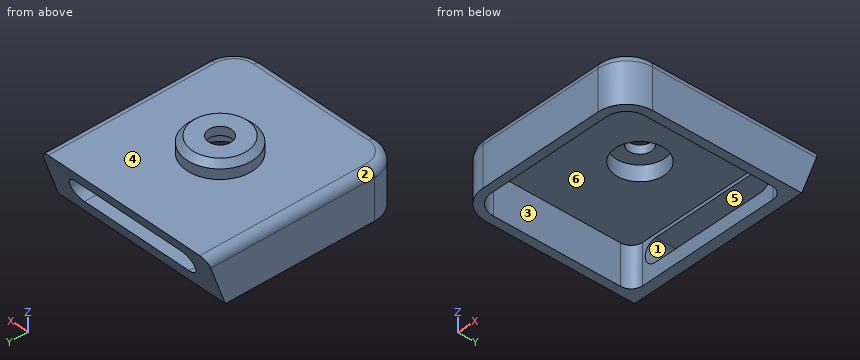
from build123d import *

# Parameters (mm, degrees)
SKETCH1_W           = 32
SKETCH1_H           = 31.091910702798558
BOSS_EXTRUDE1_DEPTH = 1.5
FILLET1_R           = 5
SKETCH2_R           = 4.3000000000159515
CUT_EXTRUDE1_DEPTH  = 45.642545975233084
SKETCH3_R           = 5.79999999998862
SKETCH3_R_2         = 4.299999999994187
BOSS_EXTRUDE2_DEPTH = 1.212999868
SKETCH4_R           = 5.799999999994187
SKETCH4_R_2         = 1.9999999999941904
BOSS_EXTRUDE3_DEPTH = 1.5
CHAMFER1_SIZE       = 1
EXTRUDE_THIN1_DEPTH = 7.05
BOSS_EXTRUDE4_REACH = 47.171
SKETCH7_W           = 29.000000000000004
SKETCH7_H           = 1.8000000000000007
BOSS_EXTRUDE5_DEPTH = 7.05
FILLET2_R           = 2
CUT_EXTRUDE2_DEPTH  = 10
FILLET3_R           = 1.5


with BuildPart() as part:
    # Sketch1 → Boss-Extrude1 (new body)
    with BuildSketch(Plane.XY):
        with Locations((16, 15.545955351399279)):
            Rectangle(SKETCH1_W, SKETCH1_H)
    extrude(amount=BOSS_EXTRUDE1_DEPTH)

    # Fillet1
    fillet1_edges = [part.edges().sort_by_distance(p)[0] for p in [
        (32, 0, 0.75),
        (0, 0, 0.75),
    ]]
    fillet(fillet1_edges, radius=FILLET1_R)

    # Sketch2 → Cut-Extrude1 (cut, through all)
    with BuildSketch(Plane(origin=(0, 0, 0), x_dir=(-1, 0, 0), z_dir=(0, 0, -1))):
        with Locations((-15.991678414180004, 17.403095514898066)):
            Circle(SKETCH2_R)
    extrude(amount=-CUT_EXTRUDE1_DEPTH, mode=Mode.SUBTRACT)

    # Sketch3 → Boss-Extrude2 (add)
    with BuildSketch(Plane.XY.offset(1.5)):
        with Locations(Location((15.991678414180004, 17.403095514898066, 0), (0, 0, 180))):
            Circle(SKETCH3_R)
        with Locations(Location((15.991678414180004, 17.403095514898066, 0), (0, 0, 180))):
            Circle(SKETCH3_R_2, mode=Mode.SUBTRACT)
    extrude(amount=BOSS_EXTRUDE2_DEPTH)

    # Sketch4 → Boss-Extrude3 (add)
    with BuildSketch(Plane.XY.offset(2.7129998678795)):
        with Locations(Location((15.991678414180004, 17.403095514898066, 0), (0, 0, 180))):
            Circle(SKETCH4_R)
        with Locations((15.991678414180004, 17.403095514898066)):
            Circle(SKETCH4_R_2, mode=Mode.SUBTRACT)
    extrude(amount=BOSS_EXTRUDE3_DEPTH)

    # Chamfer1
    chamfer1_edges = [part.edges().sort_by_distance(p)[0] for p in [
        (21.791678414174193, 17.403095514898062, 4.2129998678795),
    ]]
    chamfer(chamfer1_edges, length=CHAMFER1_SIZE)

    # Sketch5 → Extrude-Thin1 (add)
    with BuildSketch(Plane(origin=(0, 0, 0), x_dir=(-1, 0, 0), z_dir=(0, 0, -1))):
        with BuildLine():
            Line((0, 31.091910702798558), (0, 4.999999999999998))
            ThreePointArc((0, 4.999999999999998), (-1.4644660940672622, 1.4644660940672614), (-5, 0))
            Line((-5, 0), (-27, 0))
            ThreePointArc((-27, 0), (-30.535533905932738, 1.4644660940672654), (-32, 4.999999999999998))
            Line((-32, 4.999999999999998), (-32, 31.091910702798558))
            Line((-32, 31.091910702798558), (-30.5, 31.091910702798558))
            Line((-30.5, 31.091910702798558), (-30.5, 4.999999999999998))
            ThreePointArc((-30.5, 4.999999999999996), (-29.47487373415292, 2.5251262658470903), (-27.00000000000001, 1.5000000000000067))
            Line((-27, 1.5), (-5, 1.5))
            ThreePointArc((-4.999999999999999, 1.5), (-2.525126265847083, 2.5251262658470828), (-1.4999999999999996, 4.999999999999998))
            Line((-1.5, 4.999999999999998), (-1.5, 31.091910702798558))
            Line((-1.5, 31.091910702798558), (0, 31.091910702798558))
        make_face()
    extrude(amount=EXTRUDE_THIN1_DEPTH)

    # Boss-Extrude4: up to this face of the body (flat: up to its plane)
    boss_extrude4_end = Plane(part.part.faces().sort_by_distance((0, 18.045955351, -2.775))[0])
    # Sketch6 → Boss-Extrude4 (add, up to the picked face)
    with BuildSketch(Plane(origin=(32, 0, 0), x_dir=(0, 0, -1), z_dir=(1, 0, 0)), mode=Mode.PRIVATE) as boss_extrude4_sk1:
        Polygon((7.050000000000448, 31.09191070279875), (-1.4999999999999993, 34.20385620577456), (-1.5, 31.091910702798558), align=None)
    boss_extrude4_tool1 = split(extrude(boss_extrude4_sk1.sketch, amount=-BOSS_EXTRUDE4_REACH, mode=Mode.PRIVATE), bisect_by=boss_extrude4_end, keep=Keep.BOTH, mode=Mode.PRIVATE)
    add(boss_extrude4_tool1.solids().sort_by(Axis((32, 32.129226, -1.35), (-1, 0, 0)))[0])

    # Sketch7 → Boss-Extrude5 (add)
    with BuildSketch(Plane(origin=(0, 0, 0), x_dir=(-1, 0, 0), z_dir=(0, 0, -1))):
        with Locations((-16, 30.19191070279856)):
            Rectangle(SKETCH7_W, SKETCH7_H)
    extrude(amount=BOSS_EXTRUDE5_DEPTH)

    # Fillet2
    fillet2_edges = [part.edges().sort_by_distance(p)[0] for p in [
        (30.5, 29.291910702798557, -3.525),
        (1.5, 29.291910702798557, -3.525),
    ]]
    fillet(fillet2_edges, radius=FILLET2_R)

    # Sketch8 → Cut-Extrude2 (cut)
    with BuildSketch(Plane.XZ.offset(-29.291910702798557)):
        with BuildLine():
            Line((26, -4.600000000000001), (6.000000000000002, -4.600000000000004))
            ThreePointArc((6.000000000000002, -4.600000000000004), (3.9999999999999996, -2.600000000000004), (6.000000000000001, -0.6000000000000024))
            Line((6.000000000000001, -0.6000000000000024), (26, -0.6))
            ThreePointArc((26, -0.6), (28, -2.600000000000002), (26, -4.600000000000001))
        make_face()
    extrude(amount=-CUT_EXTRUDE2_DEPTH, mode=Mode.SUBTRACT)

    # Fillet3
    fillet3_edges = [part.edges().sort_by_distance(p)[0] for p in [
        (32, 19.60192810288728, 1.4999999999999996),
        (16, 0, 1.5),
        (1.4644660940672618, 1.4644660940672614, 1.5),
        (30.535533905932738, 1.4644660940672618, 1.5),
        (-4.4e-16, 19.60192810288728, 1.4999999999999996),
    ]]
    fillet(fillet3_edges, radius=FILLET3_R)


solid = part.part
The model under review builds one solid part; all positions refer to its coordinate system, in mm. Face numbers are marked on the shaded views. A direction names the side the tool comes from. Coordinates: 2 decimals unless noted, no trailing zeros. Order: outer loops, then holes, each group sorted by start corner. A loop starts at its lowest first (then second) coordinate and runs counter-clockwise, first axis right, second up. Notation, with made-up numbers: (-30, -6.5) -> (21, -6.5) arc R18 cw to (21, 9.5) -> close; hole circle Ø7 at (20.25, 33.25). An arc over 180 degrees is marked (long way). Answer in a Markdown table with one row per item.
(1) Consider section B-B (y = 26). Write out the cut boundary in (x, z).
Answers:
| item | result |
|---|---|
| outline | (0, -7.05) -> (1.5, -7.05) -> (1.5, 0) -> (30.5, 0) -> (30.5, -7.05) -> (32, -7.05) -> (32, 0) arc R1.5 ccw to (30.5, 1.5) -> (1.5, 1.5) arc R1.5 ccw to (0, 0) -> close |
(2) Consider section A-A (x = 9). Write out the cut boundary in (y, z), plus the area to 3 significant figures.
Answers:
| item | result |
|---|---|
| outline | (0, -7.05) -> (1.5, -7.05) -> (1.5, 0) -> (29.29, 0) -> (29.29, -0.6) -> (33.44, -0.6) -> (34.2, 1.5) -> (1.5, 1.5) arc R1.5 ccw to (0, 0) -> close; (29.29, -7.05) -> (31.09, -7.05) -> (31.98, -4.6) -> (29.29, -4.6) -> close |
| area | 69.0 mm² |
(3) Machinability: for the marked faces 4, 5 and 6, which of the approach directions +Z, -Z, +X, -X, +Y, -Y give a long, thin tool a straight path to every point of the face, cutting with its end or side? Answer none if there is none.
Answers:
| item | result |
|---|---|
| face 4 | +Z |
| face 5 | +Y |
| face 6 | -Z |
(4) Consider section C-C (z = -5.5). Write out the cut boundary in (x, y).
Answers:
| item | result |
|---|---|
| outline | (0, 5) arc R5 ccw to (5, 0) -> (27, 0) arc R5 ccw to (32, 5) -> (32, 31.66) -> (0, 31.66) -> close; hole (1.5, 5) arc R3.5 ccw to (5, 1.5) -> (27, 1.5) arc R3.5 ccw to (30.5, 5) -> (30.5, 27.29) arc R2 ccw to (28.5, 29.29) -> (3.5, 29.29) arc R2 ccw to (1.5, 27.29) -> close |
(5) The part is to be moulded in two halves that separate along Z. For the marked faces 1, 2 and 3, say which applies: +Z half, -Z half, draft (parallel to the pull), parting line (faces both ways), or undercut.
Answers:
| item | result |
|---|---|
| face 1 | undercut |
| face 2 | +Z half |
| face 3 | draft |
(6) Wall thickness on line 1 along X through (y, z) = (7, -3.25); line 2 along Y through (x, z) = (6.5, -0.75): over which ranges is each line inside the solid? List them lowest first.
Answers:
| item | result |
|---|---|
| line 1 | 0 to 1.5, 30.5 to 32 |
| line 2 | 0 to 1.5 |
(7) Insertion check: pin 1 (4.5 mm diameter, centred on x = 17, y = 17.5, fed in from -Z); pin 2 (8.5 mm diameter, centred on x = 21.5, y = 22, fed in from -Z); pin 3 (1.5 mm diameter, centred on x = 24.5, z = -1.5, fed in from +Y). Each pin has a flat end and moves straight along its axis. Give the tip position at first contact, or say it passes through.
Answers:
| item | result |
|---|---|
| pin 1 | z = 2.71 |
| pin 2 | z = 0 |
| pin 3 | y = 1.5 |
(8) Consider section D-D (y = 30). Write out the cut boundary in (x, z).
Answers:
| item | result |
|---|---|
| outline | (0, -7.05) -> (32, -7.05) -> (32, 0) arc R1.5 ccw to (30.5, 1.5) -> (1.5, 1.5) arc R1.5 ccw to (0, 0) -> close; hole (6, -4.6) -> (26, -4.6) arc R2 ccw to (26, -0.6) -> (6, -0.6) arc R2 ccw to start |
